Check sheet for the modelled part. Datum: model origin and axes. Units: mm. A direction names the side the tool comes from. Give positions to 0.01 mm unless a question says otherwise; leave off trailing zeros. Write each loop counter-clockwise with the first axis right and the second up, starting at its lowest first coordinate (ties: lowest second). Pieces come first, ordered by that corner, then holes. Notation, with made-up numbers: (0, 61) -> (33, 61) arc R34 cw to (33, 91) -> close; hole circle Ø5 at (52.5, 79). An arc over 180 degrees is marked (long way). Answer as a JSON object with one key per item and string values.
from build123d import *

# Parameters (mm, degrees)
SKETCH1_R           = 5.55625
BOSS_EXTRUDE1_DEPTH = 1.5875
SKETCH2_R           = 3.96875
BOSS_EXTRUDE2_DEPTH = 12.7
SKETCH3_R           = 2.38125
CUT_EXTRUDE1_DEPTH  = 15.2875


with BuildPart() as part:
    # Sketch1 → Boss-Extrude1 (new body)
    with BuildSketch(Plane.XY):
        Circle(SKETCH1_R)
    extrude(amount=BOSS_EXTRUDE1_DEPTH)

    # Sketch2 → Boss-Extrude2 (add)
    with BuildSketch(Plane(origin=(0, 0, 0), x_dir=(-1, 0, 0), z_dir=(0, 0, -1))):
        Circle(SKETCH2_R)
    extrude(amount=BOSS_EXTRUDE2_DEPTH)

    # Sketch3 → Cut-Extrude1 (cut, through all)
    with BuildSketch(Plane.XY.offset(1.5875)):
        Circle(SKETCH3_R)
    extrude(amount=-CUT_EXTRUDE1_DEPTH, mode=Mode.SUBTRACT)


solid = part.part
1. Sectioned sample at A-A, the plane x = 0. Enter the section's corners in (y, z), plus the area to 3 significant figures.
Determined:
{"outline": "(-5.56, 0) -> (-3.97, 0) -> (-3.97, -12.7) -> (-2.38, -12.7) -> (-2.38, 1.59) -> (-5.56, 1.59) -> close; (2.38, -12.7) -> (3.97, -12.7) -> (3.97, 0) -> (5.56, 0) -> (5.56, 1.59) -> (2.38, 1.59) -> close", "area": "50.4 mm^2"}
2. Sectioned sample at D-D, the plane z = -4.75. Enter the section's corners in (x, y), plus the area to 3 significant figures.
Determined:
{"outline": "circle Ø7.94 at (0, 0); hole circle Ø4.76 at (0, 0)", "area": "31.7 mm^2"}
3. Mould release check, pull along X, two halves, no side actions. Record for faces 1 (the face through (0.86, -3.874, -6.261)), 2 (the face through (1.2, -2.4, 1.588)), 3 (the face through (-1.89, -1.45, -5.46)): released by +X, released by -X, zero draft, split by the parting line, or undercut.
Determined:
{"face 1": "split by the parting line", "face 2": "zero draft", "face 3": "undercut"}
4. Scan lines: L1, parallel to Y at x = 0, z = -1.5; L2, parallel to Z at x = -4, y = -0.5; L3, parallel to Y at x = 2, z = -9.5. Record each from-to range of solid material in increasing order. Write a range as [from, to].
Determined:
{"L1": "[-3.97, -2.38], [2.38, 3.97]", "L2": "[0, 1.59]", "L3": "[-3.43, -1.29], [1.29, 3.43]"}
5. Sectioned sample at C-C, the plane x = -3. Enter the section's corners in (y, z).
Determined:
{"outline": "(-4.68, 0) -> (-2.6, 0) -> (-2.6, -12.7) -> (2.6, -12.7) -> (2.6, 0) -> (4.68, 0) -> (4.68, 1.59) -> (-4.68, 1.59) -> close"}
6. Go/stop test with flat-tipped pins: P1, Ø2, axis at x = -3, y = 4.5, coming from the -Z side; P2, Ø5, axis at x = 2, z = -3, coming from the +Y side; P3, Ø2, axis at x = 2, z = -4, coming from the -Y side. Record where each tip stops, or that it passes through.
Determined:
{"P1": "z = 0", "P2": "y = 3.97", "P3": "y = -3.84"}
7. Access from +Z, -Z, +X, -X, +Y, -Y to the whole of each face (thin tool, end or side, straight path). Record for faces 4 (the face through (-2, -2, -12.7)), 5 (the face through (-4, 1, 0)).
Determined:
{"face 4": "-Z, +X, -X, +Y, -Y", "face 5": "-Z"}
